Geometry check sheet. Reference: the model listing, model coordinates, mm. Face numbers are marked on the shaded views. A direction names the side the tool comes from. Give positions to 0.01 mm unless a question says otherwise; leave off trailing zeros. Loops run counter-clockwise (first coordinate to the right, second up) from the corner with the lowest first, then second, coordinate; pieces in that order, holes last. Notation, with made-up numbers: (76, 56) -> (87, 56) arc R11 cw to (87, 63) -> close; hole circle Ø5 at (-21, 72.25). An arc over 180 degrees is marked (long way). Answer as a JSON object with one key per item and string values.
from build123d import *

# Parameters (mm, degrees)
BOSS_EXTRUDE1_DEPTH = 6
SKETCH2_R           = 1.65
CUT_EXTRUDE1_DEPTH  = 6.5
FILLET1_R           = 4
FILLET2_R           = 3


with BuildPart() as part:
    # Sketch1 → Boss-Extrude1 (new body)
    with BuildSketch(Plane(origin=(0, 0, 0), x_dir=(1, 0, 0), z_dir=(0, 1, 0))):
        Polygon((4.7, 0), (-4.7, 0), (-8, -3.3), (-8, -4.5), (-3.85, -4.5), (-3.85, -5.5), (3.85, -5.5), (3.85, -4.5), (8, -4.5), (8, -3.3), align=None)
    extrude(amount=BOSS_EXTRUDE1_DEPTH)

    # Sketch2 → Cut-Extrude1 (cut, through all)
    with BuildSketch(Plane.XY.offset(5.5)):
        with Locations((0, 3)):
            Circle(SKETCH2_R)
    extrude(amount=-CUT_EXTRUDE1_DEPTH, mode=Mode.SUBTRACT)

    # Fillet1
    fillet1_edges = [part.edges().sort_by_distance(p)[0] for p in [
        (3.85, 0, 5),
        (-3.85, 6, 5),
    ]]
    fillet(fillet1_edges, radius=FILLET1_R)

    # Fillet2
    fillet2_edges = [part.edges().sort_by_distance(p)[0] for p in [
        (8, 0, 3.9),
        (-8, 6, 3.9),
    ]]
    fillet(fillet2_edges, radius=FILLET2_R)


solid = part.part
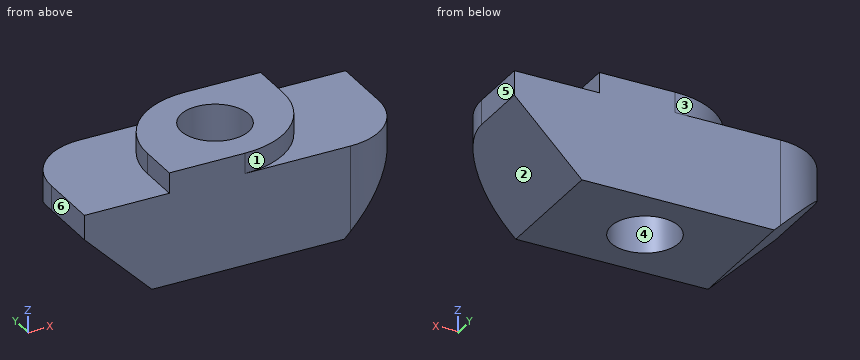
1) Section check B-B on y = 4.5. Record the cut outline in (x, z).
Geometry check:
{"outline": "(-7.6, 2.9) -> (-4.7, 0) -> (-0.69, 0) -> (-0.69, 5.5) -> (-2.97, 5.5) -> (-2.97, 4.5) -> (-7.6, 4.5) -> close; (0.69, 0) -> (4.7, 0) -> (8, 3.3) -> (8, 4.5) -> (3.85, 4.5) -> (3.85, 5.5) -> (0.69, 5.5) -> close"}
2) Tool access check on the marked faces 1, 2 and 3. Record the directions out of +Z, -Z, +X, -X, +Y, -Y that give a thin tool (end or side, any length) a straight path to the whole face; none if there is none.
Geometry check:
{"face 1": "+Z, +X, -Y", "face 2": "-Z, +X, +Y, -Y", "face 3": "+Z, -X, +Y"}
3) Section check A-A on z = 3.9. Record the cut outline in (x, y), plus the area to 3 significant figures.
Geometry check:
{"outline": "(-8, 0) -> (5, 0) arc R3 ccw to (8, 3) -> (8, 6) -> (-5, 6) arc R3 ccw to (-8, 3) -> close; hole circle Ø3.3 at (0, 3)", "area": "83.6 mm2"}
4) Section check D-D on z = 0.45. Record the cut outline in (x, y).
Geometry check:
{"outline": "(-5.15, 0) -> (5, 0) arc R3 ccw to (5.15, 0) -> (5.15, 6) -> (-5, 6) arc R3 ccw to (-5.15, 6) -> close; hole circle Ø3.3 at (0, 3)"}
5) Depth check by flat-ended pin: P1, Ø1, axis at x = 4, y = 0.5, coming from the +Z side; P2, Ø1.5, axis at x = 0, y = 5, coming from the -Z side; P3, Ø1, axis at y = 5, z = 1.5, coming from the -X side. Enter the tip coordinate at first touch or a pass-through.
Geometry check:
{"P1": "stops at z = 4.5", "P2": "stops at z = 0", "P3": "stops at x = -6.7"}
6) Material ranges on line 1 along Y through (x, z) = (0, 1.9); line 2 along Z through (x, y) = (4, 4.75); line 3 along X through (y, z) = (2.5, 2.7), recorded low to high. Write a range as from..to.
Geometry check:
{"line 1": "y = 0..1.35, 4.65..6", "line 2": "z = 0..4.5", "line 3": "x = -7.4..-1.57, 1.57..7.4"}
7) Draft check along X on the marked faces 4, 5 and 6. Enter one of: pulls with the +X half, pulls with the -X half, needs draft (parallel to the pull), parting line crosses it, or undercut.
Geometry check:
{"face 4": "undercut", "face 5": "pulls with the +X half", "face 6": "pulls with the -X half"}
